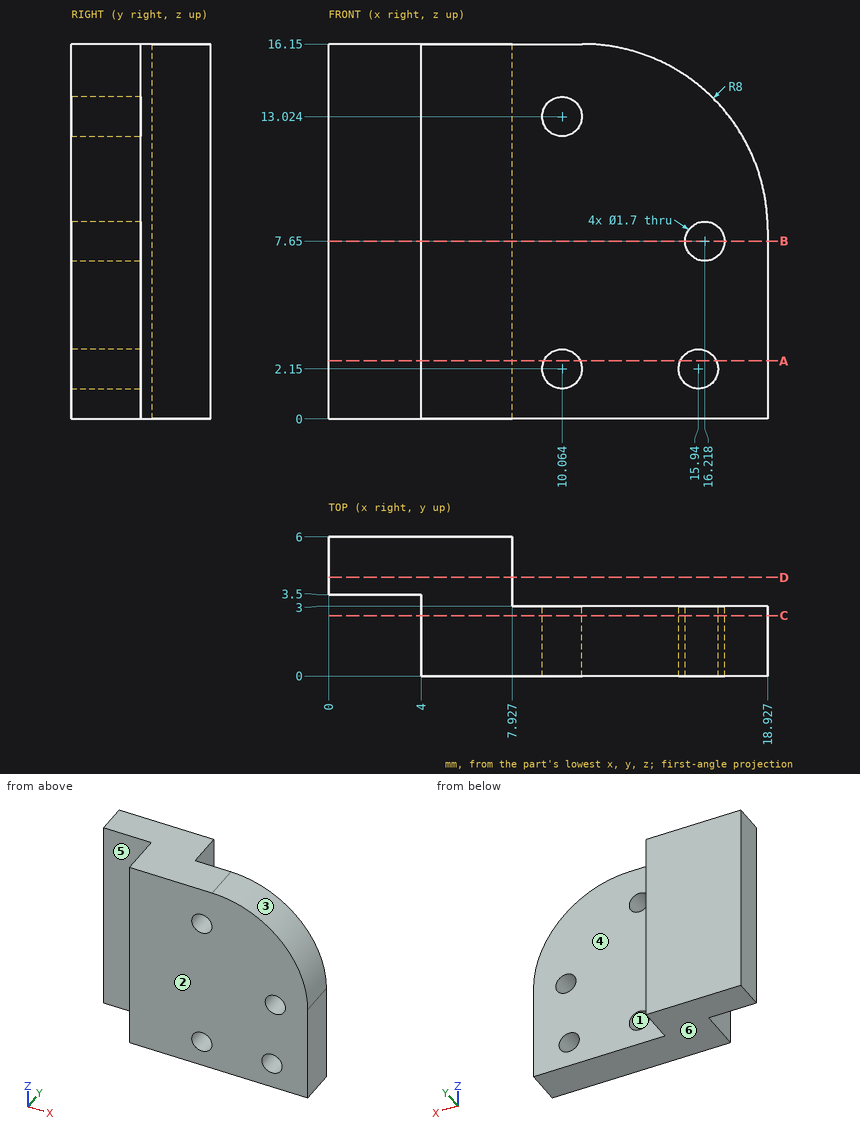
Check sheet for the drawn part. Datum: minimum x, y, z corner. Units: mm. A direction names the side the tool comes from. Coordinates: 2 decimals unless noted, no trailing zeros. Loops run counter-clockwise (first coordinate to the right, second up) from the corner with the lowest first, then second, coordinate; pieces in that order, holes last. Notation, with made-up numbers: (87.25, 78) -> (113.25, 78) arc R35 ccw to (113.25, 117) -> close; hole circle Ø5 at (46, 20). An arc over 180 degrees is marked (long way). Answer in a Markdown table with one row per item.
1) Draft check along X on the marked faces 1, 2 and 3. Enter one of: released by +X, released by -X, zero draft, split by the parting line, or undercut.
The answers:
| item | result |
|---|---|
| face 1 | undercut |
| face 2 | zero draft |
| face 3 | released by +X |
2) Section check C-C (y = 2.6). Record the cut outline in (x, z), and give its area (3 significant figures).
The answers:
| item | result |
|---|---|
| outline | (4, 0) -> (18.93, 0) -> (18.93, 8.15) arc R8 ccw to (10.93, 16.15) -> (4, 16.15) -> close; hole circle Ø1.7 at (10.06, 2.15); hole circle Ø1.7 at (10.06, 13.02); hole circle Ø1.7 at (15.94, 2.15); hole circle Ø1.7 at (16.22, 7.65) |
| area | 218 mm2 |
3) Section check B-B (z = 7.65). Record the cut outline in (x, y).
The answers:
| item | result |
|---|---|
| outline | (0, 3.5) -> (4, 3.5) -> (4, 0) -> (15.37, 0) -> (15.37, 3) -> (7.93, 3) -> (7.93, 6) -> (0, 6) -> close; (17.07, 0) -> (18.93, 0) -> (18.93, 3) -> (17.07, 3) -> close |
4) Section check A-A (z = 2.5). Record the cut outline in (x, y) (1 decimal).
The answers:
| item | result |
|---|---|
| outline | (0, 3.5) -> (4, 3.5) -> (4, 0) -> (9.3, 0) -> (9.3, 3) -> (7.9, 3) -> (7.9, 6) -> (0, 6) -> close; (10.8, 0) -> (15.2, 0) -> (15.2, 3) -> (10.8, 3) -> close; (16.7, 0) -> (18.9, 0) -> (18.9, 3) -> (16.7, 3) -> close |
5) Scan lines: line 1 along X through (y, z) = (2.15, 2.15); line 2 along X through (y, z) = (1.85, 7.65); line 3 along X through (y, z) = (2.05, 1.75) (1 decimal). Record each from-to range of solid material in increasing order. Write a range as from..to.
The answers:
| item | result |
|---|---|
| line 1 | x = 4..9.21, 10.91..15.09, 16.79..18.93 |
| line 2 | x = 4..15.37, 17.07..18.93 |
| line 3 | x = 4..9.3, 10.8..15.2, 16.7..18.9 |
6) Access from +Z, -Z, +X, -X, +Y, -Y to the whole of each face (thin tool, end or side, straight path). Record for the marked faces 4, 5 and 6.
The answers:
| item | result |
|---|---|
| face 4 | +Z, -Z, +X, +Y |
| face 5 | +Z, -Z, -X, -Y |
| face 6 | -Z, +X, -X, +Y, -Y |
7) Depth check by flat-ended pin: P1, Ø3.5, axis at y = 5, z = 6, coming from the +X side; P2, Ø5.5, axis at x = 15, z = 4.5, coming from the +Y side. Enter the tip coordinate at first touch or a pass-through.
The answers:
| item | result |
|---|---|
| P1 | stops at x = 7.93 |
| P2 | stops at y = 3 |
8) Section check D-D (y = 4.25). Record the cut outline in (x, z), and give its area (3 significant figures).
The answers:
| item | result |
|---|---|
| outline | (0, 0) -> (7.93, 0) -> (7.93, 16.15) -> (0, 16.15) -> close |
| area | 128 mm2 |
